Input: part model. Units: mm. Frame: model coordinates. Face numbers are marked on the shaded views. A direction names the side the tool comes from. Give positions to 0.01 mm unless a question says otherwise; leave off trailing zeros. Loops run counter-clockwise (first coordinate to the right, second up) from the corner with the lowest first, then second, coordinate; pieces in that order, holes last. Notation, with made-up numbers: (-20, 11) - (30, 11) arc R11 ccw to (30, 18) - close; hole circle Ø4 at (54, 35). An arc over 180 degrees is marked (long way). Answer as a JSON object with one key per item and string values.
from build123d import *

# Parameters (mm, degrees)
F1_DEPTH = 1.2
F2_R     = 5
F3_DEPTH = 1.2
F4_R     = 4
F5_DEPTH = 3


with BuildPart() as f1:
    # F0 (on Top) → F1 (new body)
    with BuildSketch(Plane.XY):
        Polygon((-11, 3.574117), (-11, -3.574117), (-6.798374, -9.357159), (0, -11.566084), (6.798374, -9.357159), (11, -3.574117), (11, 3.574117), (6.798374, 9.357159), (0, 11.566084), (-6.798374, 9.357159), align=None)
    extrude(amount=F1_DEPTH)

    # F2 (on face) → F3 (join)
    with BuildSketch(Plane.XY.offset(1.2)):
        Circle(F2_R)
    extrude(amount=F3_DEPTH)

    # F4 (on face) → F5 (join)
    with BuildSketch(Plane.XY.offset(2.4)):
        Circle(F4_R)
    extrude(amount=F5_DEPTH)


solid = f1.part
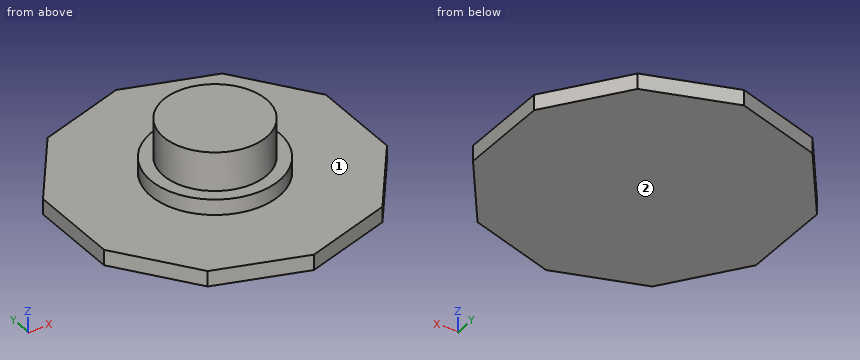
Item 1: Cut plane A-A (y = 0). Return loops of the section in (x, z), then the cut area to 3 significant figures.
Geometry check:
{"outline": "(-11, 0) - (11, 0) - (11, 1.2) - (5, 1.2) - (5, 2.4) - (4, 2.4) - (4, 5.4) - (-4, 5.4) - (-4, 2.4) - (-5, 2.4) - (-5, 1.2) - (-11, 1.2) - close", "area": "62.4 mm2"}
Item 2: Cut plane B-B (x = 1.5). Return loops of the section in (y, z), then the cut area to 3 significant figures.
Geometry check:
{"outline": "(-11.08, 0) - (11.08, 0) - (11.08, 1.2) - (4.77, 1.2) - (4.77, 2.4) - (3.71, 2.4) - (3.71, 5.4) - (-3.71, 5.4) - (-3.71, 2.4) - (-4.77, 2.4) - (-4.77, 1.2) - (-11.08, 1.2) - close", "area": "60.3 mm2"}
Item 3: Cut plane C-C (z = 4.3). Return loops of the section in (x, y), then the cut area to 3 significant figures.
Geometry check:
{"outline": "circle Ø8 at (0, 0)", "area": "50.3 mm2"}
Item 4: Material intervals for line 1 (Z direction, x = -3.5, y = -6.25); line 2 (X direction, y = 3.5, z = 2.3); line 3 (X direction, y = 3, z = 2.1), sorted ascending. Write a range as [from, to].
Geometry check:
{"line 1": "z = [0, 1.2]", "line 2": "x = [-3.57, 3.57]", "line 3": "x = [-4, 4]"}
Item 5: Contact query for flat-ended pins moving along their axis: P1, Ø3, axis at x = 8, y = -6, coming from the +Z side; P2, Ø1.5, axis at x = 4.5, y = 2.5, coming from the +Z side. Output: stop coordinate, or through.
Geometry check:
{"P1": "stops at z = 1.2", "P2": "stops at z = 2.4"}
Item 6: Access query for the marked faces 1 and 2. Directions: +Z, -Z, +X, -X, +Y, -Y. A direction counts if a zero-diameter tool reaches every point of the face in a straight line with its end or side. Return the directions, or none.
Geometry check:
{"face 1": "+Z", "face 2": "-Z, +X, -X, +Y, -Y"}
Item 7: Cut plane D-D (x = 4.5). Return loops of the section in (y, z).
Geometry check:
{"outline": "(-10.1, 0) - (10.1, 0) - (10.1, 1.2) - (2.18, 1.2) - (2.18, 2.4) - (-2.18, 2.4) - (-2.18, 1.2) - (-10.1, 1.2) - close"}
